```python
from build123d import *

# Parameters (mm, degrees)
SKETCH1_W                      = 84
SKETCH1_H                      = 60
BOSS_EXTRUDE1_DEPTH            = 15
SKETCH2_W                      = 6
SKETCH2_H                      = 60
BOSS_EXTRUDE2_DEPTH            = 32
M3_CLEARANCE_HOLE1_D           = 3.4
SKETCH7_W                      = 38
SKETCH7_H                      = 60
BOSS_EXTRUDE3_DEPTH            = 3.5
CUT_EXTRUDE5_START             = -7.147594
SKETCH26_W                     = 20
SKETCH26_H                     = 60
CUT_EXTRUDE5_DEPTH             = 7.147594
SKETCH30_W                     = 60
SKETCH30_H                     = 15
BOSS_EXTRUDE4_DEPTH            = 20
SKETCH27_W                     = 20
SKETCH27_H                     = 5
CUT_EXTRUDE6_DEPTH             = 111.653577801
FILLET1_R                      = 3
SKETCH28_R                     = 1.85
CUT_EXTRUDE7_DEPTH             = 111.653577801
CBORE_FOR_M5_SHCS2_D           = 5.5
CBORE_FOR_M5_SHCS2_CBORE_D     = 10
CBORE_FOR_M5_SHCS2_CBORE_DEPTH = 10
CHAMFER1_SIZE                  = 4
CHAMFER1_SIZE2                 = 3.356398525
CBORE_FOR_M5_SHCS3_D           = 5.5
CBORE_FOR_M5_SHCS3_CBORE_D     = 10
CBORE_FOR_M5_SHCS3_CBORE_DEPTH = 5
CUT_EXTRUDE8_DEPTH             = 4
CHAMFER2_SIZE                  = 0.5
SKETCH31_R                     = 15
CUT_EXTRUDE9_DEPTH             = 5
SKETCH32_R                     = 2.25
CUT_EXTRUDE10_DEPTH            = 112.445053726
CHAMFER3_SIZE                  = 0.5
FILLET2_R                      = 15
SKETCH33_R                     = 3
CUT_EXTRUDE11_DEPTH            = 109.074048744


with BuildPart() as part:
    # Sketch1 → Boss-Extrude1 (new body)
    with BuildSketch(Plane(origin=(0, 0, 0), x_dir=(1, 0, 0), z_dir=(0, 1, 0))):
        with Locations((42, 30)):
            Rectangle(SKETCH1_W, SKETCH1_H)
    extrude(amount=BOSS_EXTRUDE1_DEPTH)

    # Sketch2 → Boss-Extrude2 (add)
    with BuildSketch(Plane.XZ):
        with Locations((3, -30)):
            Rectangle(SKETCH2_W, SKETCH2_H)
    extrude(amount=BOSS_EXTRUDE2_DEPTH)

    # M3 Clearance Hole1 (through all)
    with Locations(Plane.ZY):
        with Locations((-42.5, -28.5), (-42.5, -3.5), (-17.5, -3.5), (-17.5, -28.5)):
            Hole(M3_CLEARANCE_HOLE1_D / 2)

    # Sketch7 → Boss-Extrude3 (add)
    with BuildSketch(Plane.XZ):
        with Locations((38, -30)):
            Rectangle(SKETCH7_W, SKETCH7_H)
    extrude(amount=BOSS_EXTRUDE3_DEPTH)

    # Sketch26 → Cut-Extrude5 (cut)
    with BuildSketch(Plane(origin=(0, 15, 0), x_dir=(1, 0, 0), z_dir=(0, 1, 0)).offset(CUT_EXTRUDE5_START)):
        with Locations((38, 30)):
            Rectangle(SKETCH26_W, SKETCH26_H)
    extrude(amount=CUT_EXTRUDE5_DEPTH, mode=Mode.SUBTRACT)

    # Sketch30 → Boss-Extrude4 (add)
    with BuildSketch(Plane.ZY):
        with Locations((-30, 7.5)):
            Rectangle(SKETCH30_W, SKETCH30_H)
    extrude(amount=BOSS_EXTRUDE4_DEPTH)

    # Sketch27 → Cut-Extrude6 (cut, through all)
    with BuildSketch(Plane(origin=(0, 7.852406202, 0), x_dir=(1, 0, 0), z_dir=(0, 1, 0))):
        with Locations((38, 7.5)):
            Rectangle(SKETCH27_W, SKETCH27_H)
        with Locations((38, 52.5)):
            Rectangle(SKETCH27_W, SKETCH27_H)
    extrude(amount=-CUT_EXTRUDE6_DEPTH, mode=Mode.SUBTRACT)

    # Fillet1
    fillet1_edges = [part.edges().sort_by_distance(p)[0] for p in [
        (38, -3.5, -5),
        (38, 7.852406202, -10),
        (38, -3.5, -55),
        (38, 7.852406202, -50),
    ]]
    fillet(fillet1_edges, radius=FILLET1_R)

    # Sketch28 → Cut-Extrude7 (cut, through all)
    with BuildSketch(Plane(origin=(0, 7.852406202, 0), x_dir=(1, 0, 0), z_dir=(0, 1, 0))):
        with Locations(Location((33, 30, 0), (0, 0, 270))):
            Circle(SKETCH28_R)
        with Locations(Location((43, 30, 0), (0, 0, 270))):
            Circle(SKETCH28_R)
    extrude(amount=-CUT_EXTRUDE7_DEPTH, mode=Mode.SUBTRACT)

    # CBORE for M5 SHCS2 (through all)
    with Locations(Plane(origin=(0, 15, 0), x_dir=(1, 0, 0), z_dir=(0, 1, 0))):
        with Locations((75, 52), (75, 8)):
            CounterBoreHole(CBORE_FOR_M5_SHCS2_D / 2, CBORE_FOR_M5_SHCS2_CBORE_D / 2, CBORE_FOR_M5_SHCS2_CBORE_DEPTH)

    # Chamfer1
    chamfer1_edges = [part.edges().sort_by_distance(p)[0] for p in [
        (84, 0, -30),
    ]]
    chamfer1_side = [part.faces().sort_by_distance(p)[0] for p in [
        (70.364021046, 0, -30),
    ]]
    chamfer(chamfer1_edges, length=CHAMFER1_SIZE, length2=CHAMFER1_SIZE2, reference=chamfer1_side[0])

    # CBORE for M5 SHCS3 (through all)
    with Locations(Plane(origin=(0, 0, 0), x_dir=(-1, 0, 0), z_dir=(0, -1, 0))):
        with Locations((-64.5, 52), (-64.5, 8), (12, 30)):
            CounterBoreHole(CBORE_FOR_M5_SHCS3_D / 2, CBORE_FOR_M5_SHCS3_CBORE_D / 2, CBORE_FOR_M5_SHCS3_CBORE_DEPTH)

    # Sketch20 → Cut-Extrude8 (cut)
    with BuildSketch(Plane(origin=(0, 15, 0), x_dir=(1, 0, 0), z_dir=(0, 1, 0))):
        Polygon((64.5, 12.618802154), (60.5, 10.309401077), (60.5, 5.690598923), (64.5, 3.381197846), (68.5, 5.690598923), (68.5, 10.309401077), align=None)
        Polygon((64.5, 47.381197846), (68.5, 49.690598923), (68.5, 54.309401077), (64.5, 56.618802154), (60.5, 54.309401077), (60.5, 49.690598923), align=None)
        Polygon((-8, 27.690598923), (-8, 32.309401077), (-12, 34.618802154), (-16, 32.309401077), (-16, 27.690598923), (-12, 25.381197846), align=None)
    extrude(amount=-CUT_EXTRUDE8_DEPTH, mode=Mode.SUBTRACT)

    # Chamfer2
    chamfer2_edges = [part.edges().sort_by_distance(p)[0] for p in [
        (84, 15, -30),
        (66, 15, -60),
        (70, 15, -8),
        (70, 15, -52),
        (66.5, 15, -11.464101615),
        (62.5, 15, -11.464101615),
        (60.5, 15, -8),
        (62.5, 15, -4.535898385),
        (66.5, 15, -4.535898385),
        (68.5, 15, -8),
        (62.5, 15, -48.535898385),
        (66.5, 15, -48.535898385),
        (68.5, 15, -52),
        (66.5, 15, -55.464101615),
        (62.5, 15, -55.464101615),
        (60.5, 15, -52),
        (-10, 15, -26.535898385),
        (-8, 15, -30),
        (-10, 15, -33.464101615),
        (-14, 15, -33.464101615),
        (-16, 15, -30),
        (-14, 15, -26.535898385),
        (66, 15, 0),
        (4, 15, -60),
        (28, 15, -30),
        (48, 15, -30),
        (-20, 15, -30),
        (4, 15, 0),
    ]]
    chamfer(chamfer2_edges, length=CHAMFER2_SIZE)

    # Sketch31 → Cut-Extrude9 (cut)
    with BuildSketch(Plane(origin=(0, 15, 0), x_dir=(1, 0, 0), z_dir=(0, 1, 0))):
        with Locations(Location((66, 30, 0), (0, 0, 270))):
            Circle(SKETCH31_R)
        with Locations(Location((10.5, 30, 0), (0, 0, 270))):
            Circle(SKETCH31_R)
    extrude(amount=-CUT_EXTRUDE9_DEPTH, mode=Mode.SUBTRACT)

    # Sketch32 → Cut-Extrude10 (cut, through all)
    with BuildSketch(Plane(origin=(0, 10, 0), x_dir=(1, 0, 0), z_dir=(0, 1, 0))):
        with Locations(Location((10.5, 30, 0), (0, 0, 270))):
            Circle(SKETCH32_R)
        with Locations(Location((66, 30, 0), (0, 0, 270))):
            Circle(SKETCH32_R)
    extrude(amount=-CUT_EXTRUDE10_DEPTH, mode=Mode.SUBTRACT)

    # Chamfer3
    chamfer3_edges = [part.edges().sort_by_distance(p)[0] for p in [
        (66, 15, -45),
        (10.5, 15, -45),
        (10.5, 10, -32.25),
        (66, 10, -32.25),
    ]]
    chamfer(chamfer3_edges, length=CHAMFER3_SIZE)

    # Fillet2
    # the kernel refuses this fillet: 15 mm, written as the material it adds along each edge
    with BuildSketch(Plane(origin=(0, 0, 0), x_dir=(-1, 0, 0), z_dir=(0, 0, -1))) as fillet2_piece_1_section:
        with BuildLine():
            CenterArc((FILLET2_R, -FILLET2_R), FILLET2_R, 90, 90)
            Line((0, -FILLET2_R), (0, 0))
            Line((0, 0), (FILLET2_R, 0))
        make_face()
    fillet2_piece_1 = extrude(amount=60, mode=Mode.PRIVATE)
    fillet2_piece_1 = fillet2_piece_1 - Plane(origin=(-12, -3.454719609, -30), x_dir=(-1, 0, 0), z_dir=(0, -1, 0)) * Cylinder(5, 180, mode=Mode.PRIVATE)
    fillet2_piece_1 = fillet2_piece_1 - Plane(origin=(-3.29371936, -3.5, -42.5), x_dir=(0, 0, -1), z_dir=(1, 0, 0)) * Cylinder(1.7, 180, mode=Mode.PRIVATE)
    fillet2_piece_1 = fillet2_piece_1 - Plane(origin=(-3.29371936, -3.5, -17.5), x_dir=(0, 0, -1), z_dir=(1, 0, 0)) * Cylinder(1.7, 180, mode=Mode.PRIVATE)
    add(fillet2_piece_1)

    # Sketch33 → Cut-Extrude11 (cut, through all)
    with BuildSketch(Plane.ZY):
        with Locations(Location((-17.5, -3.5, 0), (0, 0, 180))):
            Circle(SKETCH33_R)
        with Locations(Location((-42.5, -3.5, 0), (0, 0, 180))):
            Circle(SKETCH33_R)
    extrude(amount=CUT_EXTRUDE11_DEPTH, mode=Mode.SUBTRACT)


solid = part.part
```
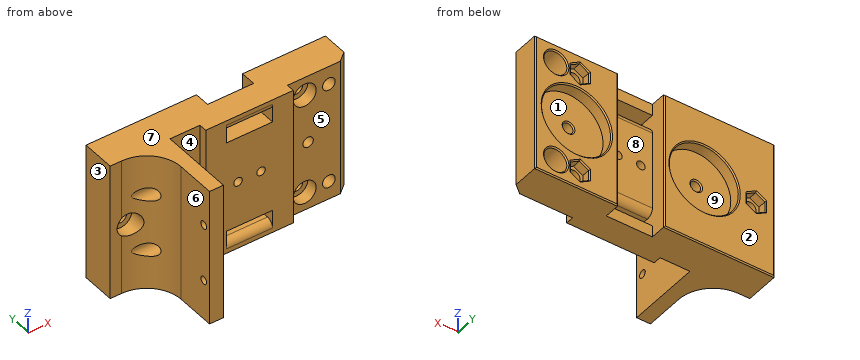
Check sheet for the modelled part. Datum: model origin and axes. Units: mm. Face numbers are marked on the shaded views. A direction names the side the tool comes from. Round coordinates to 2 decimals unless told otherwise and drop trailing zeros. Order: outer loops, then holes, each group sorted by start corner. A loop starts at its lowest first (then second) coordinate and runs counter-clockwise, first axis right, second up. Notation, with made-up numbers: (-24, -26.5) -> (-12, -26.5) arc R29 cw to (-12, 3.5) -> close; hole circle Ø5 at (-4, -19.5). An arc over 180 degrees is marked (long way). Use CSV: the item, a comma, the result in double quotes.
(1) Depth check by flat-ended pin: pin 1 (2 mm diameter, centred on y = -23.5, z = -22, fed in from -X); pin 2 (6 mm diameter, centred on x = 43, z = -30, fed in from +Y); pin 3 (2.5 mm diameter, centred on x = -16.5, z = -19, fed in from -Y). Enter the tip coordinate at first touch or a pass-through.
Worked out:
pin 1,"x = 0"
pin 2,"y = 7.85"
pin 3,"y = 0"
(2) Tool access check on the marked faces 5, 6, 7, 8 and 9. Record the directions out of +Z, -Z, +X, -X, +Y, -Y that give a thin tool (end or side, any length) a straight path to the whole face; none if there is none.
Worked out:
face 5,"+Z, -Z, +X, -Y"
face 6,"+Z, -Z, -X, -Y"
face 7,"+Z, +X, -X, +Y, -Y"
face 8,"+Z, -Z, +Y"
face 9,"+Y"
(3) Cross-section at C-C (z = -8). Count the separate pieces of the cut face and the enclosed holes in it, and give its area (3 significant figures).
Worked out:
separate pieces,"4"
enclosed holes,"0"
area,"1,310 mm²"
(4) Material ranges on line 1 along X through (y, z) = (12, -30); line 2 along Z through (x, y) = (75, 1); line 3 along X through (y, z) = (7.55, -30), recorded low to high. Write a range as from..to.
Worked out:
line 1,"-20..-16, -8..-4.5, 25.5..28, 48..51, 81..84"
line 2,"-60..-54.75, -49.25..-10.75, -5.25..0"
line 3,"-20..-14.75, -9.25..8.25, 12.75..31.15, 34.85..41.15, 44.85..63.75, 68.25..84"
(5) Draft check along X on the marked faces 1, 2, 3 and 4. Enter one of: pulls with the +X half, pulls with the -X half, needs draft (parallel to the pull), parting line crosses it, or undercut.
Worked out:
face 1,"undercut"
face 2,"needs draft"
face 3,"pulls with the -X half"
face 4,"undercut"
(6) Cross-section at D-D (y = -22.5). Record the boundary of the cut face in (x, z), and give its area (3 significant figures).
Worked out:
outline,"(0, -60) -> (6, -60) -> (6, 0) -> (0, 0) -> close"
area,"360 mm²"
(7) Cross-section at A-A (x = 43). Record the boundary of the cut face in (y, z), and give its area (3 significant figures).
Worked out:
outline,"(-3.5, -60) -> (7.85, -60) -> (7.85, -55) -> (-0.5, -55) arc R3 ccw to (-3.5, -58) -> close; (-3.5, -50) -> (4.85, -50) arc R3 ccw to (7.85, -47) -> (7.85, -31.85) -> (-3.5, -31.85) -> close; (-3.5, -28.15) -> (7.85, -28.15) -> (7.85, -13) arc R3 ccw to (4.85, -10) -> (-3.5, -10) -> close; (-3.5, -2) arc R3 ccw to (-0.5, -5) -> (7.85, -5) -> (7.85, 0) -> (-3.5, 0) -> close"
area,"518 mm²"
(8) Cross-section at B-B (y = -28.5). Record the boundary of the cut face in (x, z).
Worked out:
outline,"(0, -60) -> (6, -60) -> (6, -44.2) -> (0, -44.2) -> close; (0, -40.8) -> (6, -40.8) -> (6, -19.2) -> (0, -19.2) -> close; (0, -15.8) -> (6, -15.8) -> (6, 0) -> (0, 0) -> close"
